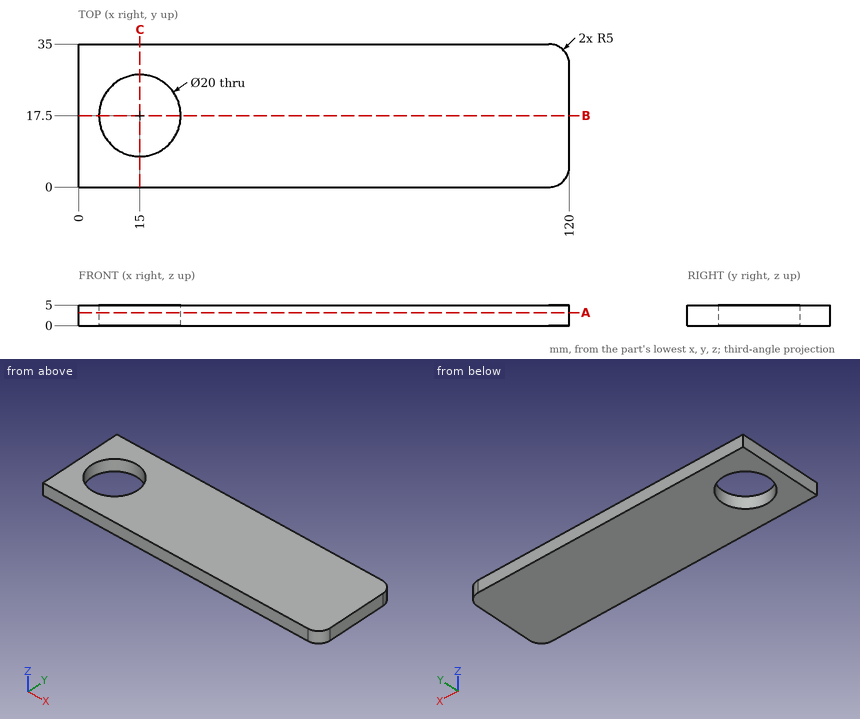
Here's the drawing with two shaded views (mm, measured from the low corner). I have some questions. Round coordinates to 2 decimals unless told otherwise and drop trailing zeros. Loops run counter-clockwise (first coordinate to the right, second up) from the corner with the lowest first, then second, coordinate; pieces in that order, holes last. Notation, with made-up numbers: (-18.75, 83.25) - (-0.75, 83.25) arc R12 ccw to (-0.75, 101.25) - close; hole circle Ø4 at (85.5, 0.5). An arc over 180 degrees is marked (long way). Write item = value, one per line.
1) Imagine slicing it at C-C (x = 15). Please give me the cut outline in (y, z), and give its area (3 significant figures).
Computed:
outline = (0, 0) - (7.5, 0) - (7.5, 5) - (0, 5) - close; (27.5, 0) - (35, 0) - (35, 5) - (27.5, 5) - close
area = 75.0 mm2
2) Imagine slicing it at A-A (z = 3.15). Please give me the cut outline in (x, y).
Computed:
outline = (0, 0) - (115, 0) arc R5 ccw to (120, 5) - (120, 30) arc R5 ccw to (115, 35) - (0, 35) - close; hole circle Ø20 at (15, 17.5)
3) Imagine slicing it at B-B (y = 17.5). Please give me the cut outline in (x, z).
Computed:
outline = (0, 0) - (5, 0) - (5, 5) - (0, 5) - close; (25, 0) - (120, 0) - (120, 5) - (25, 5) - close
4) I need wall thicknesses on line 1 along Y through (x, z) = (15, 2.35); line 2 along X through (y, z) = (19, 0.3); line 3 along Y through (x, z) = (6, 0.35). Which ranges of each line are inside material? Lowest first, please. Write a range as from..to.
Computed:
line_1 = 0..7.5, 27.5..35
line_2 = 0..5.11, 24.89..120
line_3 = 0..13.14, 21.86..35
